Read the model definition and answer for the solid it produces. Units are mm, in the model's axes. Face numbers are marked on the shaded views. A direction names the side the tool comes from. Coordinates: 2 decimals unless noted, no trailing zeros. Write each loop counter-clockwise with the first axis right and the second up, starting at its lowest first coordinate (ties: lowest second). Pieces come first, ordered by that corner, then holes. Notation, with made-up numbers: (-15.5, 77.5) - (26.5, 77.5) arc R25 cw to (26.5, 113.5) - close; hole circle Ø7 at (70.5, -8). An arc over 180 degrees is marked (long way). Return JSON: item names as keys, results as strings.
```python
from build123d import *

# Parameters (mm, degrees)
F1_DEPTH    = 8
F3_DEPTH    = 16.001
F2_R        = 1.3
F4_DEPTH    = 16.001
F2_R_2      = 1.75
F5_DEPTH    = 3.5
F6_R        = 1.3
F7_DEPTH    = 7
F8_T1_DEPTH = 19.9153161013


# Not quite as in the source:
# - a fillet or chamfer that OpenCascade refuses, or shapes differently, is made with other operations: its cross-section is extruded or revolved along the edge and cut away or added


with BuildPart() as f1:
    # F0 (on Top) → F1 (new body)
    with BuildSketch(Plane.XY):
        with BuildLine():
            Line((-4.5, 3), (-4.5, 13))
            Line((-4.5, 13), (-8, 13))
            Line((-8, 13), (-8, -0.5))
            ThreePointArc((-8, -0.5), (-6.0961940777, -5.0961940777), (-1.5, -7))
            Line((-1.5, -7), (1.5, -7))
            ThreePointArc((1.5, -7), (6.0961940777, -5.0961940777), (8, -0.5))
            Line((8, -0.5), (8, 13))
            Line((8, 13), (4.5, 13))
            Line((4.5, 13), (4.5, 3))
            ThreePointArc((4.5, 3), (3.6213203436, 0.8786796564), (1.5, 0))
            Line((1.5, 0), (-1.5, 0))
            ThreePointArc((-1.5, 0), (-3.6213203436, 0.8786796564), (-4.5, 3))
        make_face()
    extrude(amount=F1_DEPTH)

    # F2 (on face) → F3 (cut, through all)
    with BuildSketch(Plane.YZ.offset(8)):
        with BuildLine():
            ThreePointArc((13, 4), (11.8284271247, 1.1715728753), (9, 0))
            Line((9, 0), (13, 0))
            Line((13, 0), (13, 4))
        make_face()
        with BuildLine():
            ThreePointArc((9, 8), (11.8284271247, 6.8284271247), (13, 4))
            Line((13, 4), (13, 8))
            Line((13, 8), (9, 8))
        make_face()
    extrude(amount=-F3_DEPTH, mode=Mode.SUBTRACT)

    # F2 (on face) → F4 (cut, through all)
    with BuildSketch(Plane.YZ.offset(8)):
        with Locations((9, 4)):
            Circle(F2_R)
    extrude(amount=-F4_DEPTH, mode=Mode.SUBTRACT)

    # F2 (on face) → F5 (cut, through all)
    with BuildSketch(Plane.YZ.offset(8)):
        with Locations((9, 4)):
            Circle(F2_R_2)
        with Locations((9, 4)):
            Circle(F2_R, mode=Mode.SUBTRACT)
    extrude(amount=-F5_DEPTH, mode=Mode.SUBTRACT)

    # F6 (on face) → F7 (cut, through all)
    with BuildSketch(Plane(origin=(0, 0, 0), x_dir=(-1, 0, 0), z_dir=(0, 1, 0))):
        with Locations((0, 4)):
            Circle(F6_R)
    extrude(amount=-F7_DEPTH, mode=Mode.SUBTRACT)

    # F8: chamfer of 1.5 on 2 edges, made by hand

    # F8_s2 → F8_t1 (cut)
    with BuildSketch(Plane.XZ.offset(-12.8575244819)):
        Polygon((-6.5, 0), (-8, 1.5), (-8, 0), align=None)
        Polygon((-6.5, 8), (-8, 6.5), (-8, 8), align=None)
    extrude(amount=F8_T1_DEPTH, mode=Mode.SUBTRACT)


solid = f1.part
```
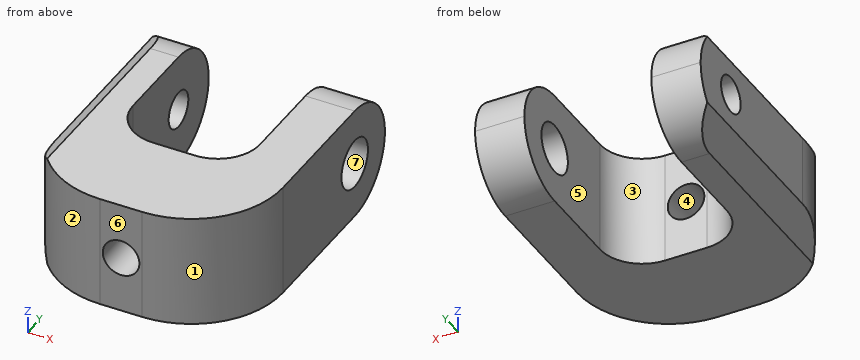
(1) Flat-ended cylindrical pins translate along their axes: P1, Ø3, axis at x = 0, z = 4, coming from the +Y side; P2, Ø1, axis at x = -5.5, y = 11, coming from the -Z side; P3, Ø2.5, axis at y = 9, z = 4, coming from the -X side; P4, Ø3, axis at x = -1.5, z = 1.5, coming from the +Y side. Find the tip coordinate at first contact, or state that the pin passes through.
Answer:
{"P1": "y = 0", "P2": "z = 0.29", "P3": "through", "P4": "y = 0.4"}
(2) Determine the mould class of the marked faces 1, 2, 3 and 4 for opening direction X: +X half, -X half, draft (parallel to the pull), parting line (faces both ways), or undercut.
Answer:
{"face 1": "+X half", "face 2": "-X half", "face 3": "undercut", "face 4": "undercut"}
(3) A cutting plane is placed at C-C (y = -3). Determine the outline of the cut face in (x, z), and give its area (3 significant figures).
Answer:
{"outline": "(-7.5, 1) - (-6.5, 0) - (7.5, 0) - (7.5, 8) - (-6.5, 8) - (-7.5, 7) - close; hole circle Ø2.6 at (0, 4)", "area": "114 mm²"}
(4) A cutting plane is placed at A-A (y = 4.5). Determine the outline of the cut face in (x, z).
Answer:
{"outline": "(-8, 1.5) - (-6.5, 0) - (-4.5, 0) - (-4.5, 8) - (-6.5, 8) - (-8, 6.5) - close; (4.5, 0) - (8, 0) - (8, 8) - (4.5, 8) - close"}
(5) Which of the six approach directions +Z, -Z, +X, -X, +Y, -Y give full straight-line access (tool end or side, diameter ignored) to the marked faces 5, 6 and 7?
Answer:
{"face 5": "+Z, -Z, +Y", "face 6": "+Z, -Z, +X, -X, -Y", "face 7": "+X"}
(6) Straight lines are drawn through the part: line 1 (Z direction, x = 0, y = -2.25); line 2 (Z direction, x = 6.25, y = 9); line 3 (Y direction, x = 1.25, z = 7.5). For each, find the intervals that lie inside material, in ascending order. Write a range as from..to.
Answer:
{"line 1": "0..2.7, 5.3..8", "line 2": "0..2.25, 5.75..8", "line 3": "-7..0"}
(7) A cutting plane is placed at D-D (y = 8.25). Determine the outline of the cut face in (x, z).
Answer:
{"outline": "(-8, 1.5) - (-6.5, 0) - (-4.5, 0) - (-4.5, 2.94) - (-8, 2.94) - close; (-8, 5.06) - (-4.5, 5.06) - (-4.5, 8) - (-6.5, 8) - (-8, 6.5) - close; (4.5, 0) - (8, 0) - (8, 2.42) - (4.5, 2.42) - close; (4.5, 5.58) - (8, 5.58) - (8, 8) - (4.5, 8) - close"}
(8) A cutting plane is placed at B-B (x = 0). Determine the outline of the cut face in (y, z), and give its area (3 significant figures).
Answer:
{"outline": "(-7, 0) - (0, 0) - (0, 2.7) - (-7, 2.7) - close; (-7, 5.3) - (0, 5.3) - (0, 8) - (-7, 8) - close", "area": "37.8 mm²"}
